Work out the finished part from the listing and answer in its coordinate system (mm). Coordinates: 2 decimals unless noted, no trailing zeros. Order: outer loops, then holes, each group sorted by start corner. A loop starts at its lowest first (then second) coordinate and runs counter-clockwise, first axis right, second up. Notation, with made-up numbers: M 29.5,-40 L 85.5,-40 A5 cw 85.5,-34 Z; hole C 85.5,-12.75 d3. An arc over 180 degrees is marked long. Use a Markdown table: item, result.
from build123d import *

# Parameters (mm, degrees)
SKETCH1_W           = 76.2
SKETCH1_H           = 88.9
BOSS_EXTRUDE1_DEPTH = 6.35
SKETCH2_R           = 2.0193
SKETCH2_W           = 50.8
SKETCH2_H           = 19.05
CUT_EXTRUDE1_DEPTH  = 6.35
SKETCH3_W           = 6.35
SKETCH3_H           = 9.525
SKETCH3_W_2         = 9.525
SKETCH3_H_2         = 6.35
BOSS_EXTRUDE3_DEPTH = 6.35


with BuildPart() as part:
    # Sketch1 → Boss-Extrude1 (new body)
    with BuildSketch(Plane.XY):
        with Locations((38.1, -44.45)):
            Rectangle(SKETCH1_W, SKETCH1_H)
    extrude(amount=BOSS_EXTRUDE1_DEPTH)

    # Sketch2 → Cut-Extrude1 (cut)
    with BuildSketch(Plane.XY.offset(6.35)):
        with Locations((51.9176, -9.652)):
            Circle(SKETCH2_R)
        with Locations((51.9176, -38.608)):
            Circle(SKETCH2_R)
        with Locations((24.2824, -38.6842)):
            Circle(SKETCH2_R)
        with Locations((24.2824, -9.652)):
            Circle(SKETCH2_R)
        with BuildLine():
            Line((48.26, 0), (48.26, -38.1))
            ThreePointArc((48.26, -38.1), (38.1, -48.26), (27.94, -38.1))
            Line((27.94, -38.1), (27.94, 0))
            ThreePointArc((27.94, 0), (38.1, 10.16), (48.26, 0))
        make_face()
        with Locations((38.1, -73.025)):
            Rectangle(SKETCH2_W, SKETCH2_H)
    extrude(amount=-CUT_EXTRUDE1_DEPTH, mode=Mode.SUBTRACT)

    # Sketch3 → Boss-Extrude3 (add)
    with BuildSketch(Plane.XY):
        with Locations((-3.175, -14.2875)):
            Rectangle(SKETCH3_W, SKETCH3_H)
        with Locations((-3.175, -33.3375)):
            Rectangle(SKETCH3_W, SKETCH3_H)
        with Locations((-3.175, -52.3875)):
            Rectangle(SKETCH3_W, SKETCH3_H)
        with Locations((-3.175, -71.4375)):
            Rectangle(SKETCH3_W, SKETCH3_H)
        with Locations((4.7625, -92.075)):
            Rectangle(SKETCH3_W_2, SKETCH3_H_2)
        with Locations((23.8125, -92.075)):
            Rectangle(SKETCH3_W_2, SKETCH3_H_2)
        with Locations((42.8625, -92.075)):
            Rectangle(SKETCH3_W_2, SKETCH3_H_2)
        with Locations((61.9125, -92.075)):
            Rectangle(SKETCH3_W_2, SKETCH3_H_2)
        with Locations((79.375, -71.4375)):
            Rectangle(SKETCH3_W, SKETCH3_H)
        with Locations((79.375, -52.3875)):
            Rectangle(SKETCH3_W, SKETCH3_H)
        with Locations((79.375, -33.3375)):
            Rectangle(SKETCH3_W, SKETCH3_H)
        with Locations((79.375, -14.2875)):
            Rectangle(SKETCH3_W, SKETCH3_H)
    extrude(amount=BOSS_EXTRUDE3_DEPTH)


solid = part.part
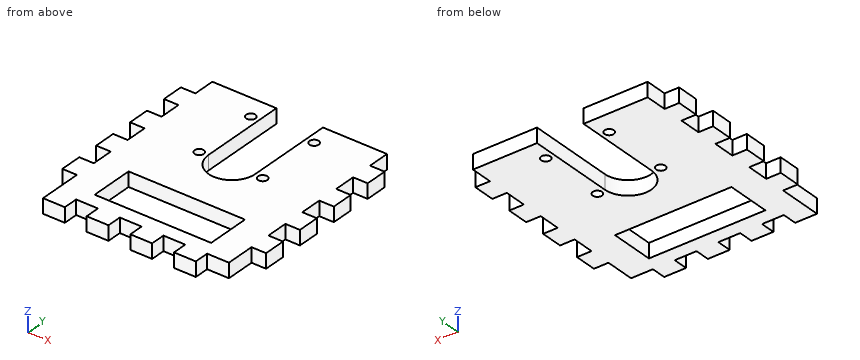
(1) A cutting plane is placed at C-C (z = 3.75). Give the number of separate pieces and of enclosed holes in the cut face, then the cut area to 3 significant figures.
Conclusion:
| item | result |
|---|---|
| separate pieces | 1 |
| enclosed holes | 5 |
| area | 5,540 mm2 |
(2) Straight lines are drawn through the part: L1, parallel to Y at x = -2, z = 4.5 (3 decimals); L2, parallel to X at y = -72.5, z = 1.75; L3, parallel to X at y = -80, z = 1.5. For each, find the intervals that lie inside material, in ascending order.
Conclusion:
| item | result |
|---|---|
| L1 | -76.2 to -66.675, -57.15 to -47.625, -38.1 to -28.575, -19.05 to -9.525 |
| L2 | -6.35 to 12.7, 63.5 to 82.55 |
| L3 | 0 to 12.7, 63.5 to 76.2 |
(3) A cutting plane is placed at B-B (x = 17). Determine the outline of the cut face in (y, z), then the cut area to 3 significant figures.
Conclusion:
| item | result |
|---|---|
| outline | M -88.9,0 L -82.55,0 L -82.55,6.35 L -88.9,6.35 Z; M -63.5,0 L 0,0 L 0,6.35 L -63.5,6.35 Z |
| area | 444 mm2 |
(4) Given P1, Ø2, axis at y = -84.5, z = 1.5, coming from the +X side; P2, Ø1.9, axis at x = 80.5, z = 5, coming from the -Y side; P3, Ø3, axis at x = 31.5, z = 4.5, coming from the -Y side, each flat-ended and moving along its own axis, determine where each tip first touches the part or whether it passes through.
Conclusion:
| item | result |
|---|---|
| P1 | x = 76.2 |
| P2 | y = -76.2 |
| P3 | y = -88.9 |
(5) A cutting plane is placed at A-A (y = -68.5). Determine the outline of the cut face in (x, z).
Conclusion:
| item | result |
|---|---|
| outline | M -6.35,0 L 12.7,0 L 12.7,6.35 L -6.35,6.35 Z; M 63.5,0 L 82.55,0 L 82.55,6.35 L 63.5,6.35 Z |
